Verification items for the finished model (mm, model axes). A direction names the side the tool comes from. Give positions to 0.01 mm unless a question says otherwise; leave off trailing zeros. Order: outer loops, then holes, each group sorted by start corner. A loop starts at its lowest first (then second) coordinate and runs counter-clockwise, first axis right, second up. Notation, with made-up numbers: (-3, -24) - (38, -24) arc R17 ccw to (38, -16) - close; hole circle Ø8 at (85, 14). An arc over 180 degrees is marked (long way). Answer as a JSON object with one key per item and string values.
```python
from build123d import *

# Parameters (mm, degrees)
SKETCH1_W           = 51.308
SKETCH1_H           = 80.518
BOSS_EXTRUDE1_DEPTH = 5.334
SKETCH2_W           = 5.334
SKETCH2_H           = 16.1036
CUT_EXTRUDE1_DEPTH  = 57.679185374
SKETCH3_W           = 4.318
SKETCH3_H           = 5.334
CUT_EXTRUDE2_DEPTH  = 57.679185374


with BuildPart() as part:
    # Sketch1 → Boss-Extrude1 (new body)
    with BuildSketch(Plane.XY):
        with Locations((-13.293278732, 0.572213281)):
            Rectangle(SKETCH1_W, SKETCH1_H)
    extrude(amount=BOSS_EXTRUDE1_DEPTH)

    # Sketch2 → Cut-Extrude1 (cut, through all)
    with BuildSketch(Plane.XY.offset(5.334)):
        with Locations((-36.280278732, 16.675813281)):
            Rectangle(SKETCH2_W, SKETCH2_H)
        with Locations((-36.280278732, -15.531386719)):
            Rectangle(SKETCH2_W, SKETCH2_H)
        with Locations((9.693721268, -15.531386719)):
            Rectangle(SKETCH2_W, SKETCH2_H)
        with Locations((9.693721268, 16.675813281)):
            Rectangle(SKETCH2_W, SKETCH2_H)
    extrude(amount=-CUT_EXTRUDE1_DEPTH, mode=Mode.SUBTRACT)

    # Sketch3 → Cut-Extrude2 (cut, through all)
    with BuildSketch(Plane.XY.offset(5.334)):
        with Locations((-22.564278732, 38.164213281)):
            Rectangle(SKETCH3_W, SKETCH3_H)
        with Locations((4.867721268, 38.164213281)):
            Rectangle(SKETCH3_W, SKETCH3_H)
    extrude(amount=-CUT_EXTRUDE2_DEPTH, mode=Mode.SUBTRACT)


solid = part.part
```
(1) Section check C-C (x = 5). Record the cut outline in (y, z), then the cut area to 3 significant figures.
Computed values:
{"outline": "(-39.69, 0) - (35.5, 0) - (35.5, 5.33) - (-39.69, 5.33) - close", "area": "401 mm²"}
(2) Section check B-B (y = 20). Record the cut outline in (x, z).
Computed values:
{"outline": "(-33.61, 0) - (7.03, 0) - (7.03, 5.33) - (-33.61, 5.33) - close"}
(3) Gauge pin test, flat ends, axial feed: pin 1 Ø2.5 at (y, z) = (-15.5, 2.5) entering from -X; pin 2 Ø2 at (x, z) = (4.5, 2.5) entering from +Y. Record the tip position at first contact, or that the pin passes through.
Computed values:
{"pin 1": "stops at x = -33.61", "pin 2": "stops at y = 35.5"}
(4) Material ranges on line 1 along Y through (x, z) = (10, 1.8); line 2 along X through (y, z) = (18.5, 1); line 3 along Y through (x, z) = (-23, 2.6), recorded low to high. Write a range as [from, to].
Computed values:
{"line 1": "y = [-39.69, -23.58], [-7.48, 8.62], [24.73, 40.83]", "line 2": "x = [-33.61, 7.03]", "line 3": "y = [-39.69, 35.5]"}
(5) Release check for a two-part mould opening along X. For faces 1 (the flat face through (-23, 35.497, 3)), 2 (the flat face through (7.027, 17, 3)), 3 (the flat face through (-20.405, 38, 3)), 4 (the flat face through (-36, 8.624, 3)) record: pulls with the +X half, pulls with the -X half, needs draft (parallel to the pull), parting line crosses it, or undercut.
Computed values:
{"face 1": "undercut", "face 2": "pulls with the +X half", "face 3": "undercut", "face 4": "needs draft"}
(6) Access from +Z, -Z, +X, -X, +Y, -Y to the whole of each face (thin tool, end or side, straight path). Record for faces 5 (the flat face through (-36, -7.48, 3)), 6 (the flat face through (10, 40.831, 3)), 7 (the flat face through (10, -7.48, 3)), 8 (the flat face through (7.027, 38, 3)), 9 (the flat face through (12.361, -32, 3)).
Computed values:
{"face 5": "+Z, -Z, -X", "face 6": "+Z, -Z, +X, -X, +Y", "face 7": "+Z, -Z, +X", "face 8": "+Z, -Z, +Y", "face 9": "+Z, -Z, +X, +Y, -Y"}
(7) Section check A-A (z = 1.05). Record the cut outline in (x, y), then the cut area to 3 significant figures.
Computed values:
{"outline": "(-38.95, -39.69) - (12.36, -39.69) - (12.36, -23.58) - (7.03, -23.58) - (7.03, -7.48) - (12.36, -7.48) - (12.36, 8.62) - (7.03, 8.62) - (7.03, 24.73) - (12.36, 24.73) - (12.36, 40.83) - (7.03, 40.83) - (7.03, 35.5) - (2.71, 35.5) - (2.71, 40.83) - (-20.41, 40.83) - (-20.41, 35.5) - (-24.72, 35.5) - (-24.72, 40.83) - (-38.95, 40.83) - (-38.95, 24.73) - (-33.61, 24.73) - (-33.61, 8.62) - (-38.95, 8.62) - (-38.95, -7.48) - (-33.61, -7.48) - (-33.61, -23.58) - (-38.95, -23.58) - close", "area": "3,740 mm²"}
